```python
from build123d import *

# Parameters (mm, degrees)
F2_R     = 1.5
F3_DEPTH = 12.5


with BuildPart() as f1:
    # F0 (on Front) → F1 (revolve)
    with BuildSketch(Plane.XZ):
        Polygon((1.145912, 0), (0, 0), (0, -6.25), (1, -6.25), (1, -7), (15, -7), (15, -6.2), (11.016158, -4.75), (4, -4.75), align=None)
    revolve(axis=Axis((0.572956, 0, 0), (-1, 0, 0)))

    # F2 (on Front) → F3 (cut, symmetric)
    with BuildSketch(Plane.XZ):
        with Locations((8, 0)):
            Circle(F2_R)
    extrude(amount=F3_DEPTH, both=True, mode=Mode.SUBTRACT)


solid = f1.part
```
The model under review builds one solid part; all positions refer to its coordinate system, in mm. A direction names the side the tool comes from. Give positions to 0.01 mm unless a question says otherwise; leave off trailing zeros. Write each loop counter-clockwise with the first axis right and the second up, starting at its lowest first coordinate (ties: lowest second). Pieces come first, ordered by that corner, then holes. Notation, with made-up numbers: (27, -6.75) - (67, -6.75) arc R25 ccw to (67, 24.25) - close; hole circle Ø4 at (51, 38). An arc over 180 degrees is marked (long way). Answer in a Markdown table with one row per item. Add a question column.
1. We need section D-D on x = 13.75. Write out the cut boundary in (y, z), then the cut area to 3 significant figures.
2. We need section B-B on z = -0.5. State how many separate pieces and enclosed holes the cut face has, then the cut area to 3 significant figures.
3. Wall thickness on line 1 along Z through (x, y) = (6.75, 0); line 2 along Z through (x, y) = (2.75, 3.25): over which ranges is each line inside the solid? List them lowest first. Write a range as [from, to].
4. Draft analysis for pull direction Y (two halves, no side actions). For faces 1 (the cylindrical face through (0.51, -1.88, -5.96)), 2 (the conical face through (11.21, -1.448, -4.598)), 3 (the cylindrical face through (7.805, -5.767, 1.487)), state which applies: +Y half, -Y half, draft (parallel to the pull), parting line (faces both ways), or undercut.
5. Tool access review of faces 4 (the flat face through (0, 0, 0)), 5 (the cylindrical face through (7.459, 1.819, -4.388)), 6 (the flat face through (1, -6, -3)): name each direction out of +Z, -Z, +X, -X, +Y, -Y from which nothing blocks a thin tool from reaching the whole face with its end or side.
6. We need section C-C on x = 5.25. Write out the cut boundary in (y, z).
7. Insertion check: P1, Ø4, axis at x = 9, z = 5, coming from the +Y side; P2, Ø1, axis at x = 3.5, y = 5, coming from the +Z side. Each pin has a flat end and moves straight along its axis. Give the tip position at first contact, or say it passes through.
8. We need section A-A on x = 8. Write out the cut boundary in (y, z).
Ans:
| question | item | result |
|---|---|---|
| 1 | outline | circle Ø14 at (0, 0); hole circle Ø11.49 at (0, 0) |
| 1 | area | 50.2 mm^2 |
| 2 | separate pieces | 3 |
| 2 | enclosed holes | 0 |
| 2 | area | 72.4 mm^2 |
| 3 | line 1 | z = [-7, -4.75], [4.75, 7] |
| 3 | line 2 | z = [-6.2, 6.2] |
| 4 | face 1 | parting line |
| 4 | face 2 | undercut |
| 4 | face 3 | draft |
| 5 | face 4 | +Z, -Z, -X, +Y, -Y |
| 5 | face 5 | +X |
| 5 | face 6 | -X |
| 6 | outline | circle Ø14 at (0, 0); hole circle Ø9.5 at (0, 0) |
| 7 | P1 | stops at y = 6.32 |
| 7 | P2 | stops at z = 5.36 |
| 8 | outline | (-6.84, -1.5) arc R7 ccw to (6.84, -1.5) - (4.51, -1.5) arc R4.75 cw to (-4.51, -1.5) - close; (-6.84, 1.5) - (-4.51, 1.5) arc R4.75 cw to (4.51, 1.5) - (6.84, 1.5) arc R7 ccw to start |
